```python
from build123d import *

# Parameters (mm, degrees)
SKETCH1_W           = 60
SKETCH1_H           = 23
BOSS_EXTRUDE1_DEPTH = 3
BOSS_EXTRUDE2_DEPTH = 3
SKETCH3_R           = 1
CUT_EXTRUDE1_DEPTH  = 88.299770905
FILLET1_R           = 2


with BuildPart() as part:
    # Sketch1 → Boss-Extrude1 (new body)
    with BuildSketch(Plane.XY):
        Rectangle(SKETCH1_W, SKETCH1_H)
    extrude(amount=BOSS_EXTRUDE1_DEPTH)

    # Sketch2 → Boss-Extrude2 (add)
    with BuildSketch(Plane.XY.offset(3)):
        Polygon((50, 11.5), (-50, 11.5), (-50, 71.5), (-30, 71.5), (-30, 31.5), (30, 31.5), (30, 71.5), (50, 71.5), align=None)
    extrude(amount=-BOSS_EXTRUDE2_DEPTH)

    # Sketch3 → Cut-Extrude1 (cut, through all)
    with BuildSketch(Plane.XY.offset(3)):
        with Locations((-30, 11.5)):
            Circle(SKETCH3_R)
        with Locations((30, 11.5)):
            Circle(SKETCH3_R)
    extrude(amount=-CUT_EXTRUDE1_DEPTH, mode=Mode.SUBTRACT)

    # Fillet1
    fillet1_edges = [part.edges().sort_by_distance(p)[0] for p in [
        (50, 11.5, 1.5),
        (-50, 11.5, 1.5),
        (30, -11.5, 1.5),
        (-30, -11.5, 1.5),
    ]]
    fillet(fillet1_edges, radius=FILLET1_R)


solid = part.part
```
Work out the finished part from the listing and answer in its coordinate system (mm). A direction names the side the tool comes from. Round coordinates to 2 decimals unless told otherwise and drop trailing zeros. Loops run counter-clockwise (first coordinate to the right, second up) from the corner with the lowest first, then second, coordinate; pieces in that order, holes last. Notation, with made-up numbers: (42, 30.25) -> (65, 30.25) arc R7 ccw to (65, 41.25) -> close; hole circle Ø6 at (54, 27). An arc over 180 degrees is marked (long way). Write each question's results on one line, items separated by ' | '. Start each with the question number.
1. Given pin 1 Ø1.5 at (x, z) = (15, 1.5) entering from +Y, flat-ended and moving along its own axis, determine where the tip first touches the part or whether it passes through.
2. A tool of negligible diameter and unlimited length cuts with its end or side. For faces 4 (the face through (-39, 11.5, 2)), 5 (the face through (30, 0, 1)), 6 (the face through (0, 31.5, 2)), from which of +Z, -Z, +X, -X, +Y, -Y can it reach the whole face along a straight path? Write none if from no direction.
3. Find the intervals of material crossed by probe 1 along X at (y, z) = (62, 2.2); probe 2 along Y at (x, z) = (11.5, 1.85); probe 3 along Y at (x, z) = (33, 1.7), in increasing order. Write a range as from..to.
4. Section B-B (z = 1.1) is taken. Determine the outline of the cut face in (x, y), plus the area to 3 significant figures.
5. Section D-D (y = -6) is taken. Determine the outline of the cut face in (x, z), plus the area to 3 significant figures.
6. Section A-A (y = 36) is taken. Determine the outline of the cut face in (x, z), plus the area to 3 significant figures.
7. Section C-C (x = -16) is taken. Determine the outline of the cut face in (y, z).
8. For a pull along X with two mould halves and no side action, classify faces 1 (the face through (50, 43, 2)), 2 (the face through (-29.27, 12.183, 1.521)), 3 (the face through (40, 11.5, 2)) as +X half, -X half, draft (parallel to the pull), parting line (faces both ways), or undercut.
Evaluation:
1) pin 1: stops at y = 31.5
2) face 4: +Z, -Z, -X, -Y | face 5: +Z, -Z, +X, -Y | face 6: +Z, -Z, +Y
3) probe 1: x = -50..-30, 30..50 | probe 2: y = -11.5..31.5 | probe 3: y = 11.5..71.5
4) outline: (-50, 13.5) arc R2 ccw to (-48, 11.5) -> (-31, 11.5) arc R1 cw (long way) to (-30, 10.5) -> (-30, -9.5) arc R2 ccw to (-28, -11.5) -> (28, -11.5) arc R2 ccw to (30, -9.5) -> (30, 10.5) arc R1 cw (long way) to (31, 11.5) -> (48, 11.5) arc R2 ccw to (50, 13.5) -> (50, 71.5) -> (30, 71.5) -> (30, 31.5) -> (-30, 31.5) -> (-30, 71.5) -> (-50, 71.5) -> close | area: 4,970 mm2
5) outline: (-30, 0) -> (30, 0) -> (30, 3) -> (-30, 3) -> close | area: 180 mm2
6) outline: (-50, 0) -> (-30, 0) -> (-30, 3) -> (-50, 3) -> close; (30, 0) -> (50, 0) -> (50, 3) -> (30, 3) -> close | area: 120 mm2
7) outline: (-11.5, 0) -> (31.5, 0) -> (31.5, 3) -> (-11.5, 3) -> close
8) face 1: +X half | face 2: undercut | face 3: draft
